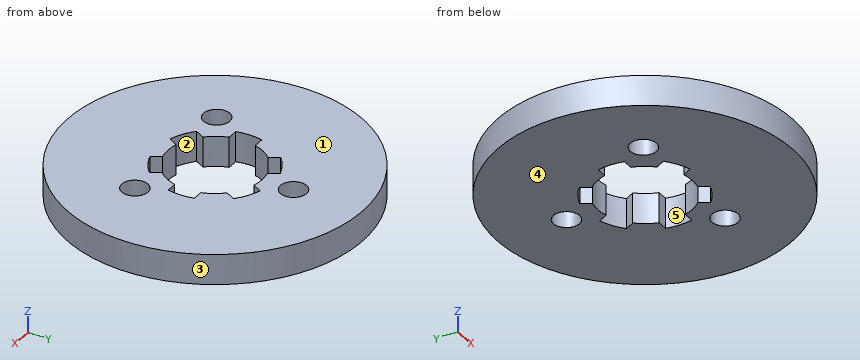
```python
from build123d import *

# Parameters (mm, degrees)
SKETCH1_R           = 28.173882667
SKETCH1_R_2         = 2.5
BOSS_EXTRUDE1_DEPTH = 5.7658


with BuildPart() as part:
    # Sketch1 → Boss-Extrude1 (new body)
    with BuildSketch(Plane.XY):
        with Locations(Location((0, 0, 0), (0, 0, 180))):
            Circle(SKETCH1_R)
        with Locations(Location((0, 15, 0), (0, 0, 180))):
            Circle(SKETCH1_R_2, mode=Mode.SUBTRACT)
        with Locations(Location((12.990381057, -7.5, 0), (0, 0, 180))):
            Circle(SKETCH1_R_2, mode=Mode.SUBTRACT)
        with Locations(Location((-12.990381057, -7.5, 0), (0, 0, 180))):
            Circle(SKETCH1_R_2, mode=Mode.SUBTRACT)
        with BuildLine():
            Line((-10.712142643, 2.5), (-8.645808233, 2.5))
            ThreePointArc((-8.645808233, 2.5), (-7.794228634, 4.5), (-6.487967626, 6.237489566))
            Line((-6.487967626, 6.237489566), (-7.521134831, 8.026987658))
            ThreePointArc((-7.521134831, 8.026987658), (-5.5, 9.526279442), (-3.191007812, 10.526987658))
            Line((-3.191007812, 10.526987658), (-2.157840607, 8.737489566))
            ThreePointArc((-2.157840607, 8.737489566), (0, 9), (2.157840607, 8.737489566))
            Line((2.157840607, 8.737489566), (3.191007812, 10.526987658))
            ThreePointArc((3.191007812, 10.526987658), (5.5, 9.526279442), (7.521134831, 8.026987658))
            Line((7.521134831, 8.026987658), (6.487967626, 6.237489566))
            ThreePointArc((6.487967626, 6.237489566), (7.794228634, 4.5), (8.645808233, 2.5))
            Line((8.645808233, 2.5), (10.712142643, 2.5))
            ThreePointArc((10.712142643, 2.5), (11, 0), (10.712142643, -2.5))
            Line((10.712142643, -2.5), (8.645808233, -2.5))
            ThreePointArc((8.645808233, -2.5), (7.794228634, -4.5), (6.487967626, -6.237489566))
            Line((6.487967626, -6.237489566), (7.521134831, -8.026987658))
            ThreePointArc((7.521134831, -8.026987658), (5.5, -9.526279442), (3.191007812, -10.526987658))
            Line((3.191007812, -10.526987658), (2.157840607, -8.737489566))
            ThreePointArc((2.157840607, -8.737489566), (0, -9), (-2.157840607, -8.737489566))
            Line((-2.157840607, -8.737489566), (-3.191007812, -10.526987658))
            ThreePointArc((-3.191007812, -10.526987658), (-5.5, -9.526279442), (-7.521134831, -8.026987658))
            Line((-7.521134831, -8.026987658), (-6.487967626, -6.237489566))
            ThreePointArc((-6.487967626, -6.237489566), (-7.794228634, -4.5), (-8.645808233, -2.5))
            Line((-8.645808233, -2.5), (-10.712142643, -2.5))
            ThreePointArc((-10.712142643, -2.5), (-11, 0), (-10.712142643, 2.5))
        make_face(mode=Mode.SUBTRACT)
    extrude(amount=BOSS_EXTRUDE1_DEPTH)


solid = part.part
```
Geometry check sheet. Reference: the model listing, model coordinates, mm. Face numbers are marked on the shaded views. A direction names the side the tool comes from. Coordinates: 2 decimals unless noted, no trailing zeros. Order: outer loops, then holes, each group sorted by start corner. A loop starts at its lowest first (then second) coordinate and runs counter-clockwise, first axis right, second up. Notation, with made-up numbers: (-23, -5.75) - (6, -5.75) arc R20 ccw to (6, 13.25) - close; hole circle Ø10 at (49, 13.25). An arc over 180 degrees is marked (long way). Answer as a JSON object with one key per item and string values. Group by question number.
Item 1: Depth check by flat-ended pin: pin 1 Ø1 at (x, z) = (-10, 1.5) entering from -Y; pin 2 Ø1.5 at (x, z) = (-20.5, 3) entering from -Y; pin 3 Ø1.7 at (x, z) = (9.5, 3.5) entering from +Y; pin 4 Ø3 at (x, y) = (12.99, -7.5) entering from +Z. Enter the tip coordinate at first touch or a pass-through.
Item 2: Tool access check on the marked faces 4 and 5. Record the directions out of +Z, -Z, +X, -X, +Y, -Y that give a thin tool (end or side, any length) a straight path to the whole face; none if there is none.
Item 3: Sectioned sample at A-A, the plane x = 0. Record the cut outline in (y, z).
Item 4: Draft check along X on the marked faces 1, 2 and 3. Enter one of: +X half, -X half, draft (parallel to the pull), parting line (faces both ways), or undercut.
Item 5: Scan lines: probe 1 along Y at (x, z) = (0, 3.05); probe 2 along Y at (x, z) = (-1, 3.5); probe 3 along X at (y, z) = (-7.5, 4.2). Record each from-to range of solid material in increasing order.
Item 6: Sectioned sample at C-C, the plane y = 15. Record the cut outline in (x, z), and give its area (3 significant figures).
Item 7: Sectioned sample at D-D, the plane y = 4.5. Record the cut outline in (x, z), and give its area (3 significant figures).
Item 8: Sectioned sample at B-B, the plane z = 2.4. Record the cut outline in (x, y).
Resolved:
{
 "1": {"pin 1": "y = -26.52", "pin 2": "y = -20.09", "pin 3": "y = 26.81", "pin 4": "through"},
 "2": {"face 4": "-Z, +X, -X, +Y, -Y", "face 5": "+Z, -Z"},
 "3": {"outline": "(-28.17, 0) - (-9, 0) - (-9, 5.77) - (-28.17, 5.77) - close; (9, 0) - (12.5, 0) - (12.5, 5.77) - (9, 5.77) - close; (17.5, 0) - (28.17, 0) - (28.17, 5.77) - (17.5, 5.77) - close"},
 "4": {"face 1": "draft", "face 2": "undercut", "face 3": "parting line"},
 "5": {"probe 1": "-28.17 to -9, 9 to 12.5, 17.5 to 28.17", "probe 2": "-28.16 to -8.94, 8.94 to 12.71, 17.29 to 28.16", "probe 3": "-27.16 to -15.49, -10.49 to -7.22, 7.22 to 10.49, 15.49 to 27.16"},
 "6": {"outline": "(-23.85, 0) - (-2.5, 0) - (-2.5, 5.77) - (-23.85, 5.77) - close; (2.5, 0) - (23.85, 0) - (23.85, 5.77) - (2.5, 5.77) - close", "area": "246 mm^2"},
 "7": {"outline": "(-27.81, 0) - (-7.79, 0) - (-7.79, 5.77) - (-27.81, 5.77) - close; (7.79, 0) - (27.81, 0) - (27.81, 5.77) - (7.79, 5.77) - close", "area": "231 mm^2"},
 "8": {"outline": "circle Ø56.35 at (0, 0); hole circle Ø5 at (-12.99, -7.5); hole (-10.71, -2.5) - (-8.65, -2.5) arc R9 ccw to (-6.49, -6.24) - (-7.52, -8.03) arc R11 ccw to (-3.19, -10.53) - (-2.16, -8.74) arc R9 ccw to (2.16, -8.74) - (3.19, -10.53) arc R11 ccw to (7.52, -8.03) - (6.49, -6.24) arc R9 ccw to (8.65, -2.5) - (10.71, -2.5) arc R11 ccw to (10.71, 2.5) - (8.65, 2.5) arc R9 ccw to (6.49, 6.24) - (7.52, 8.03) arc R11 ccw to (3.19, 10.53) - (2.16, 8.74) arc R9 ccw to (-2.16, 8.74) - (-3.19, 10.53) arc R11 ccw to (-7.52, 8.03) - (-6.49, 6.24) arc R9 ccw to (-8.65, 2.5) - (-10.71, 2.5) arc R11 ccw to start; hole circle Ø5 at (0, 15); hole circle Ø5 at (12.99, -7.5)"}
}
